Read the model definition and answer for the solid it produces. Units are mm, in the model's axes. Coordinates: 2 decimals unless noted, no trailing zeros. Loops run counter-clockwise (first coordinate to the right, second up) from the corner with the lowest first, then second, coordinate; pieces in that order, holes last. Notation, with made-up numbers: (-4.75, 74.25) -> (41.25, 74.25) arc R20 ccw to (41.25, 104.25) -> close; hole circle Ø3 at (14.25, 9). An arc over 180 degrees is marked (long way). Answer as a JSON object with one key per item and string values. Group by question number.
Q1. The part is cut by section A-A on x = 2. Write down the section's boundary in (y, z).
Q2. Determine the mould class of faces 1 (the cylindrical face through (0, 13, 14)), 2 (the cylindrical face through (0, 14, -13)), 3 (the cylindrical face through (-0.04, 11.52, 8.34)), 4 (the cylindrical face through (-0.04, -8.48, 8.34)) for opening direction Z: released by +Z, released by -Z, zero draft, split by the parting line, or undercut.
Q3. The part is cut by section B-B on y = 0. Write down the section's boundary in (x, z) (3 decimals), and give its area (3 significant figures).
Q4. The part is cut by section C-C on z = -4. Write down the section's boundary in (x, y) (3 decimals), and give its area (3 significant figures).
Q5. The part is cut by section D-D on y = -11. Write down the section's boundary in (x, z) (3 decimals).
Q6. Straight lines are drawn through the part: line 1 along Y through (x, z) = (0.25, 10); line 2 along Z through (x, y) = (-2, 10.75); line 3 along Z through (x, y) = (-3, -11.25). For each, find the intervals that lie inside material, in ascending order. Write a range as [from, to].
from build123d import *

# Parameters (mm, degrees)
CROQUIS1_W                   = 30
CROQUIS1_H                   = 30
CROQUIS1_R                   = 9
SALIENTE_EXTRUIR1_DEPTH      = 3.175
TALADRO_DE_MARGEN_PARA_M41_D = 4.5
REDONDEO1_R                  = 5


with BuildPart() as part:
    # Croquis1 → Saliente-Extruir1 (new, symmetric)
    with BuildSketch(Plane(origin=(0, 0, 0), x_dir=(0, 0, -1), z_dir=(1, 0, 0))):
        Rectangle(CROQUIS1_W, CROQUIS1_H)
        Circle(CROQUIS1_R, mode=Mode.SUBTRACT)
    extrude(amount=SALIENTE_EXTRUIR1_DEPTH, both=True)

    # Taladro de margen para M41 (through all)
    with Locations(Plane(origin=(3.175, 0, 0), x_dir=(0, 0, -1), z_dir=(1, 0, 0))):
        with Locations((-10, 10), (-10, -10), (10, -10), (10, 10)):
            Hole(TALADRO_DE_MARGEN_PARA_M41_D / 2)

    # Redondeo1
    redondeo1_edges = [part.edges().sort_by_distance(p)[0] for p in [
        (0, -15, -15),
        (0, -15, 15),
        (0, 15, 15),
        (0, 15, -15),
    ]]
    fillet(redondeo1_edges, radius=REDONDEO1_R)


solid = part.part
Final values:
{
 "1": {"outline": "(-15, -10) arc R5 ccw to (-10, -15) -> (10, -15) arc R5 ccw to (15, -10) -> (15, 10) arc R5 ccw to (10, 15) -> (-10, 15) arc R5 ccw to (-15, 10) -> close; hole circle Ø4.5 at (-10, -10); hole circle Ø4.5 at (-10, 10); hole circle Ø18 at (0, 0); hole circle Ø4.5 at (10, -10); hole circle Ø4.5 at (10, 10)"},
 "2": {"face 1": "released by +Z", "face 2": "released by -Z", "face 3": "undercut", "face 4": "undercut"},
 "3": {"outline": "(-3.175, -15) -> (3.175, -15) -> (3.175, -9) -> (-3.175, -9) -> close; (-3.175, 9) -> (3.175, 9) -> (3.175, 15) -> (-3.175, 15) -> close", "area": "76.2 mm2"},
 "4": {"outline": "(-3.175, -15) -> (3.175, -15) -> (3.175, -8.062) -> (-3.175, -8.062) -> close; (-3.175, 8.062) -> (3.175, 8.062) -> (3.175, 15) -> (-3.175, 15) -> close", "area": "88.1 mm2"},
 "5": {"outline": "(-3.175, -14.899) -> (3.175, -14.899) -> (3.175, -12.016) -> (-3.175, -12.016) -> close; (-3.175, -7.984) -> (3.175, -7.984) -> (3.175, 7.984) -> (-3.175, 7.984) -> close; (-3.175, 12.016) -> (3.175, 12.016) -> (3.175, 14.899) -> (-3.175, 14.899) -> close"},
 "6": {"line 1": "y = [-15, -12.25], [-7.75, 7.75], [12.25, 15]", "line 2": "z = [-14.94, -12.12], [-7.88, 7.88], [12.12, 14.94]", "line 3": "z = [-14.84, -11.87], [-8.13, 8.13], [11.87, 14.84]"}
}
